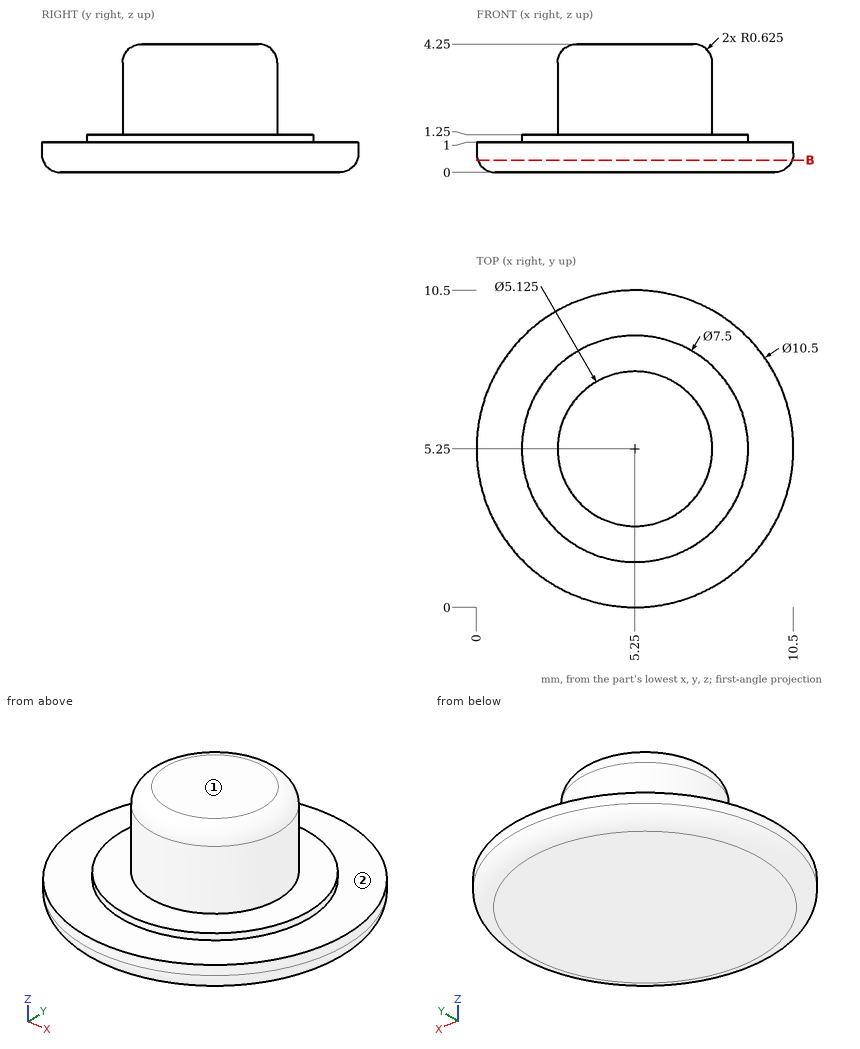
Part print with two shaded views. Sizes in mm from the minimum x, y, z corner. A direction names the side the tool comes from. Round coordinates to 2 decimals unless told otherwise and drop trailing zeros. Write each loop counter-clockwise with the first axis right and the second up, starting at its lowest first coordinate (ties: lowest second). Pieces come first, ordered by that corner, then holes. Notation, with made-up numbers: M 63.25,34 L 69.25,34 A9 cw 69.25,39 Z; hole C -24.75,-36 d6. An arc over 180 degrees is marked long. Use CSV: the item, a comma, the result in double quotes.
1. Wall check: probe 1 along Z at (x, y) = (1.75, 7.5); probe 2 along Z at (x, y) = (8, 6.75); probe 3 along X at (y, z) = (4, 1.15). Give the ranges that are in metal, low to high. Write a range as from..to.
Reply:
probe 1,"z = 0..1"
probe 2,"z = 0..1.25"
probe 3,"x = 1.71..8.79"
2. Saw through at B-B (z = 0.4). Give the cut face in (x, y).
Reply:
outline,"C 5.25,5.25 d10.42"
3. Flat gauge pins, fed straight in: pin 1 (1.5 mm diameter, centred on y = 3.5, z = 1.5, fed in from -X); pin 2 (1 mm diameter, centred on x = 6.5, z = 3.5, fed in from -Y). Where does each tip first touch, or does it go through?
Reply:
pin 1,"stops at x = 0.14"
pin 2,"stops at y = 2.8"
4. Tool access for the marked faces 1 and 2: list every direction of +Z, -Z, +X, -X, +Y, -Y with a clear straight run to the whole face (end or side of a thin tool).
Reply:
face 1,"+Z, +X, -X, +Y, -Y"
face 2,"+Z"
